Part model, mm, in its own coordinate system. A direction names the side the tool comes from. Coordinates: 2 decimals unless noted, no trailing zeros. Order: outer loops, then holes, each group sorted by start corner. A loop starts at its lowest first (then second) coordinate and runs counter-clockwise, first axis right, second up.
1) Cut at B-B (x = -2.5). List the corners of the cut face in (y, z), and give its area (3 significant figures).
2) Pin check, flat tips, straight feed: pin 1 Ø20 at (x, y) = (48, 11.5) entering from +Z; pin 2 Ø5 at (x, z) = (61, -4.5) entering from -Y; pin 3 Ø2.5 at (x, y) = (-2, 13) entering from -Z. Stop position of each tip, or through.
3) Cut at C-C (x = 43). List the corners of the cut face in (y, z), and give its area (3 significant figures).
4) Wall check: L1, parallel to Y at x = 18, z = -0.5; L2, parallel to X at y = 19.5, z = 3; L3, parallel to Z at x = 62.5, y = 12.5. Give the ranges that are in metal, low to high.
5) Tool access for faces 1 (the flat face through (49, 20, 5)), 2 (the flat face through (-2, 20, -2.5)), 3 (the flat face through (-5, 20, 5)), 4 (the flat face through (39, 0, 0)), 5 (the flat face through (49, 20, -5)): list every direction of +Z, -Z, +X, -X, +Y, -Y with a clear straight run to the whole face (end or side of a thin tool).
6) Cut at A-A (y = 32.5). List the corners of the cut face in (x, z), and give its area (3 significant figures).
```python
from build123d import *

# Parameters (mm, degrees)
BOSS_EXTRUDE1_DEPTH      = 40
SKETCH3_W                = 100
SKETCH3_H                = 40
BOSS_EXTRUDE2_DEPTH      = 5
BOSS_EXTRUDE2_DEPTH_BACK = 5
SKETCH4_W                = 10
SKETCH4_H                = 10
BOSS_EXTRUDE3_DEPTH      = 20
BOSS_EXTRUDE3_TAPER      = 7


with BuildPart() as part:
    # Sketch2 → Boss-Extrude1 (new body)
    with BuildSketch(Plane(origin=(0, 0, 0), x_dir=(1, 0, 0), z_dir=(0, 1, 0))):
        Polygon((-10, 7.5), (-10, -7.5), (-5, -7.5), (-5, -2.5), (0, -2.5), (0, 2.5), (-5, 2.5), (-5, 7.5), align=None)
    extrude(amount=BOSS_EXTRUDE1_DEPTH)

    # Sketch3 → Boss-Extrude2 (add, two sides)
    with BuildSketch(Plane.XY) as boss_extrude2_sk:
        with Locations((50, 20)):
            Rectangle(SKETCH3_W, SKETCH3_H)
    extrude(amount=BOSS_EXTRUDE2_DEPTH)
    extrude(boss_extrude2_sk.sketch, amount=-BOSS_EXTRUDE2_DEPTH_BACK)

    # Sketch4 → Boss-Extrude3 (add)
    with BuildSketch(Plane.XZ):
        with Locations((95, 0)):
            Rectangle(SKETCH4_W, SKETCH4_H)
    extrude(amount=BOSS_EXTRUDE3_DEPTH, taper=BOSS_EXTRUDE3_TAPER)


solid = part.part
```
Geometry check:
1. outline: (0, -2.5) - (40, -2.5) - (40, 2.5) - (0, 2.5) - close
1. area: 200 mm2
2. pin 1: stops at z = 5
2. pin 2: stops at y = 0
2. pin 3: stops at z = -2.5
3. outline: (0, -5) - (40, -5) - (40, 5) - (0, 5) - close
3. area: 400 mm2
4. L1: y = 0 to 40
4. L2: x = -10 to -5, 0 to 100
4. L3: z = -5 to 5
5. face 1: +Z, +X, +Y, -Y
5. face 2: -Z, +Y, -Y
5. face 3: +Z, +Y, -Y
5. face 4: +Z, -Z, -X, -Y
5. face 5: -Z, +X, +Y, -Y
6. outline: (-10, -7.5) - (-5, -7.5) - (-5, -2.5) - (0, -2.5) - (0, -5) - (100, -5) - (100, 5) - (0, 5) - (0, 2.5) - (-5, 2.5) - (-5, 7.5) - (-10, 7.5) - close
6. area: 1,100 mm2
